from build123d import *

# Parameters (mm, degrees)
EXTRUDE_THIN1_DEPTH = 10
FILLET2_R           = 3
SKETCH2_R           = 1.5
CUT_EXTRUDE1_DEPTH  = 10
SKETCH3_R           = 0.75
CUT_EXTRUDE2_DEPTH  = 10


with BuildPart() as part:
    # Sketch1 → Extrude-Thin1 (new, symmetric)
    with BuildSketch(Plane.XY):
        Polygon((0, 8), (0, 0), (-12, 0), (-12, -2), (2, -2), (2, 8), align=None)
    extrude(amount=EXTRUDE_THIN1_DEPTH, both=True)

    # Fillet2
    fillet2_edges = [part.edges().sort_by_distance(p)[0] for p in [
        (-12, -1, 10),
        (-12, -1, -10),
        (1, 8, -10),
        (1, 8, 10),
    ]]
    fillet(fillet2_edges, radius=FILLET2_R)

    # Sketch2 → Cut-Extrude1 (cut)
    with BuildSketch(Plane(origin=(0, 0, 0), x_dir=(1, 0, 0), z_dir=(0, 1, 0))):
        with Locations(Location((-8.729026119, 6, 0), (0, 0, 180))):
            Circle(SKETCH2_R)
        with Locations(Location((-8.729026119, -6, 0), (0, 0, 180))):
            Circle(SKETCH2_R)
    extrude(amount=-CUT_EXTRUDE1_DEPTH, mode=Mode.SUBTRACT)

    # Sketch3 → Cut-Extrude2 (cut)
    with BuildSketch(Plane.ZY):
        with Locations((0, 6)):
            Circle(SKETCH3_R)
    extrude(amount=-CUT_EXTRUDE2_DEPTH, mode=Mode.SUBTRACT)


solid = part.part
Check sheet for the modelled part. Datum: model origin and axes. Units: mm. A direction names the side the tool comes from. Round coordinates to 2 decimals unless told otherwise and drop trailing zeros. Loops run counter-clockwise (first coordinate to the right, second up) from the corner with the lowest first, then second, coordinate; pieces in that order, holes last. Notation, with made-up numbers: (-11.5, 68) -> (7.5, 68) arc R24 ccw to (7.5, 95) -> close; hole circle Ø7 at (-34.75, -15.75). An arc over 180 degrees is marked (long way). Put each result on its own line as item: value. Start each with the question number.
1. Section check B-B (x = -9.25). Enter the section's corners in (y, z), plus the area to 3 significant figures.
2. Section check D-D (z = -6). Enter the section's corners in (x, y).
3. Gauge pin test, flat ends, axial feed: pin 1 (2 mm diameter, centred on y = 5, z = -5.5, fed in from -X); pin 2 (6 mm diameter, centred on x = -3.5, z = -5, fed in from +Y); pin 3 (0.9 mm diameter, centred on y = 6, z = 0, fed in from -X). Record the tip position at first contact, or that the pin passes through.
4. Section check C-C (y = 6). Enter the section's corners in (x, z), plus the area to 3 significant figures.
5. Scan lines: probe 1 along Y at (x, z) = (1.35, 0); probe 2 along Z at (x, y) = (-9.5, -1); probe 3 along Y at (x, z) = (-2.75, 8.25). Record each from-to range of solid material in increasing order.
6. Draft check along X on faces 1 (the face through (-2, -1, -10)), 2 (the face through (2, 3, 0)), 3 (the face through (-7.23, -0.99, -5.93)). Enter one of: +X half, -X half, draft (parallel to the pull), parting line (faces both ways), or undercut.
7. Section check A-A (z = 0). Enter the section's corners in (x, y).
8. Access from +Z, -Z, +X, -X, +Y, -Y to the whole of each face (thin tool, end or side, straight path). Record for faces 4 (the face through (-12, -1, 0)), 5 (the face through (-6, 0, 0)).
Findings:
1. outline: (-2, -9.99) -> (0, -9.99) -> (0, -7.41) -> (-2, -7.41) -> close; (-2, -4.59) -> (0, -4.59) -> (0, 4.59) -> (-2, 4.59) -> close; (-2, 7.41) -> (0, 7.41) -> (0, 9.99) -> (-2, 9.99) -> close
1. area: 28.7 mm^2
2. outline: (-12, -2) -> (-10.23, -2) -> (-10.23, 0) -> (-12, 0) -> close; (-7.23, -2) -> (2, -2) -> (2, 8) -> (0, 8) -> (0, 0) -> (-7.23, 0) -> close
3. pin 1: stops at x = 0
3. pin 2: stops at y = 0
3. pin 3: passes through
4. outline: (0, -9.83) -> (2, -9.83) -> (2, -0.75) -> (0, -0.75) -> close; (0, 0.75) -> (2, 0.75) -> (2, 9.83) -> (0, 9.83) -> close
4. area: 36.3 mm^2
5. probe 1: y = -2 to 5.25, 6.75 to 8
5. probe 2: z = -9.96 to -7.29, -4.71 to 4.71, 7.29 to 9.96
5. probe 3: y = -2 to 0
6. face 1: draft
6. face 2: +X half
6. face 3: undercut
7. outline: (-12, -2) -> (2, -2) -> (2, 5.25) -> (0, 5.25) -> (0, 0) -> (-12, 0) -> close; (0, 6.75) -> (2, 6.75) -> (2, 8) -> (0, 8) -> close
8. face 4: +Z, -Z, -X, +Y, -Y
8. face 5: +Z, -Z, -X, +Y
